The listing builds one solid part. Answer for the finished solid, in the listing's coordinates (mm). Coordinates: 2 decimals unless noted, no trailing zeros. Order: outer loops, then holes, each group sorted by start corner. A loop starts at its lowest first (then second) coordinate and runs counter-clockwise, first axis right, second up. Notation, with made-up numbers: (55.25, 31) - (98.25, 31) arc R17 ccw to (98.25, 49) - close; hole circle Ø9 at (80.5, 89.5). An arc over 180 degrees is marked (long way). Use a Markdown table: item, result. Add a question column.
Item 1: Find the intervals of material crossed by line 1 along Z through (x, y) = (-69, -4.55); line 2 along Z through (x, y) = (-70, -0.7); line 3 along Z through (x, y) = (34, -4.5), in increasing order.
Item 2: The part is cut by section C-C, the plane x = -47. Give the vertices of the cut face in (y, z).
Item 3: The part is cut by section B-B, the plane y = -3.1. State how many separate pieces and enclosed holes the cut face has, then the cut area to 3 significant figures.
Item 4: The part is cut by section D-D, the plane z = -105.5. Give the vertices of the cut face in (x, y), then the cut area to 3 significant figures.
Item 5: Flat-ended cylindrical pins translate along their axes: P1, Ø1.5, axis at y = -1.5, z = -58.5, coming from the +X side; P2, Ø1, axis at y = -3.5, z = -80.5, coming from the +X side. Find the tip coordinate at first contact, or state that the pin passes through.
Item 6: The part is cut by section A-A, the plane x = 0. Give the vertices of the cut face in (y, z).
from build123d import *

# Parameters (mm, degrees)
F0_R     = 125
F0_R_2   = 3.5
F1_DEPTH = 5


with BuildPart() as f1:
    # F0 (on Front) → F1 (new body)
    with BuildSketch(Plane.XZ):
        Circle(F0_R)
        with Locations((-71.701327, -89.91062)):
            Circle(F0_R_2, mode=Mode.SUBTRACT)
        with Locations((25.589907, -112.11671)):
            Circle(F0_R_2, mode=Mode.SUBTRACT)
        with Locations((103.61142, -49.89663)):
            Circle(F0_R_2, mode=Mode.SUBTRACT)
        with Locations((-115, 0)):
            Circle(F0_R_2, mode=Mode.SUBTRACT)
        with Locations((-71.701327, 89.91062)):
            Circle(F0_R_2, mode=Mode.SUBTRACT)
        with BuildLine():
            ThreePointArc((-99.728162, 7.368421), (-70.710678, 70.710678), (-7.368421, 99.728162))
            ThreePointArc((-7.368421, 99.728162), (0, 100), (7.368421, 99.728162))
            ThreePointArc((7.368421, 99.728162), (70.710678, 70.710678), (99.728162, 7.368421))
            ThreePointArc((99.728162, 7.368421), (99.932017, 3.686717), (100, 0))
            ThreePointArc((100, 0), (99.932017, -3.686717), (99.728162, -7.368421))
            ThreePointArc((99.728162, -7.368421), (70.710678, -70.710678), (7.368421, -99.728162))
            ThreePointArc((7.368421, -99.728162), (0, -100), (-7.368421, -99.728162))
            ThreePointArc((-7.368421, -99.728162), (-70.710678, -70.710678), (-99.728162, -7.368421))
            ThreePointArc((-99.728162, -7.368421), (-100, 0), (-99.728162, 7.368421))
        make_face(mode=Mode.SUBTRACT)
        with Locations((103.61142, 49.89663)):
            Circle(F0_R_2, mode=Mode.SUBTRACT)
        with Locations((25.589907, 112.11671)):
            Circle(F0_R_2, mode=Mode.SUBTRACT)
    extrude(amount=F1_DEPTH)


solid = f1.part
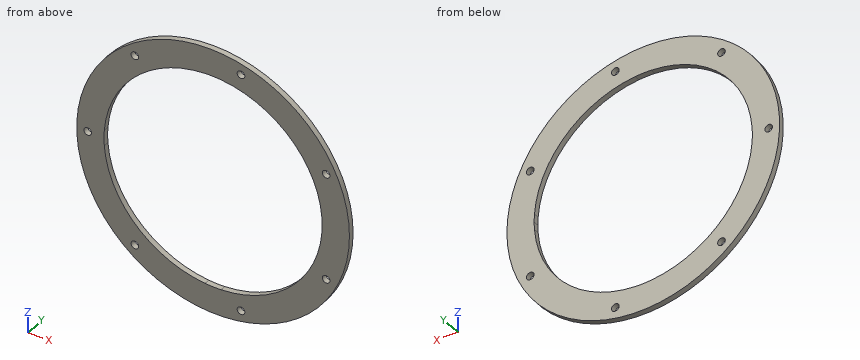
Solution:
| question | item | result |
|---|---|---|
| 1 | line 1 | z = -104.23 to -92.14, -87.69 to -72.38, 72.38 to 87.69, 92.14 to 104.23 |
| 1 | line 2 | z = -103.56 to -92.97, -86.85 to -71.41, 71.41 to 86.85, 92.97 to 103.56 |
| 1 | line 3 | z = -120.29 to -94.04, 94.04 to 120.29 |
| 2 | outline | (-5, -115.83) - (0, -115.83) - (0, -88.27) - (-5, -88.27) - close; (-5, 88.27) - (0, 88.27) - (0, 115.83) - (-5, 115.83) - close |
| 3 | separate pieces | 1 |
| 3 | enclosed holes | 8 |
| 3 | area | 17,400 mm2 |
| 4 | outline | (-67.04, -5) - (67.04, -5) - (67.04, 0) - (-67.04, 0) - close |
| 4 | area | 670 mm2 |
| 5 | P1 | stops at x = 110.86 |
| 5 | P2 | stops at x = 96.05 |
| 6 | outline | (-5, -125) - (0, -125) - (0, -100) - (-5, -100) - close; (-5, 100) - (0, 100) - (0, 125) - (-5, 125) - close |
